The drawing under review shows one solid part. Ordinate dimensions are in mm from its lowest x, y, z. A direction names the side the tool comes from. Give positions to 0.01 mm unless a question says otherwise; leave off trailing zeros. Order: outer loops, then holes, each group sorted by start corner. A loop starts at its lowest first (then second) coordinate and runs counter-clockwise, first axis right, second up. Notation, with made-up numbers: (11, -18.5) -> (58, -18.5) arc R12 ccw to (58, -1.5) -> close; hole circle Ø4 at (3.5, -26.75). An arc over 180 degrees is marked (long way). Return JSON: item names as keys, results as strings. Group by question number.
1) To check wall thickness, follow line 1 along X through (y, z) = (1.75, 1.2); line 2 along X through (y, z) = (3.5, 1.5); line 3 along Z through (x, y) = (23.25, 4.25). State the ranges of each line that lie inside material, in increasing order.
2) The part is to be moulded in two halves that separate along X. For the marked faces 1, 2 and 3, say which applies: released by +X, released by -X, zero draft, split by the parting line, or undercut.
3) Add section D-D (y = 2). State how many separate pieces and enclosed holes the cut face has, then the cut area to 3 significant figures.
4) Insertion check: P1, Ø1.5, axis at x = 24.5, y = 5, coming from the +Z side; P2, Ø2, axis at x = 10.5, z = 1, coming from the -Y side (3 decimals); P3, Ø1.5, axis at x = 21, y = 5, coming from the +Z side. Each pin has a flat end and moves straight along its axis. Give the tip position at first contact, or say it passes through.
5) Add section B-B (z = 0.95). Give the boundary of the cut face in (x, y).
6) Add section A-A (x = 25.72). Give the boundary of the cut face in (y, z).
7) Add section C-C (y = 0.5). Give the boundary of the cut face in (x, z).
8) For the marked faces 4 and 5, list the 3-axis set-ups (+Z, -Z, +X, -X, +Y, -Y) from which the entire face can be reached by the end or side of a thin tool; tool diameter is ignored.
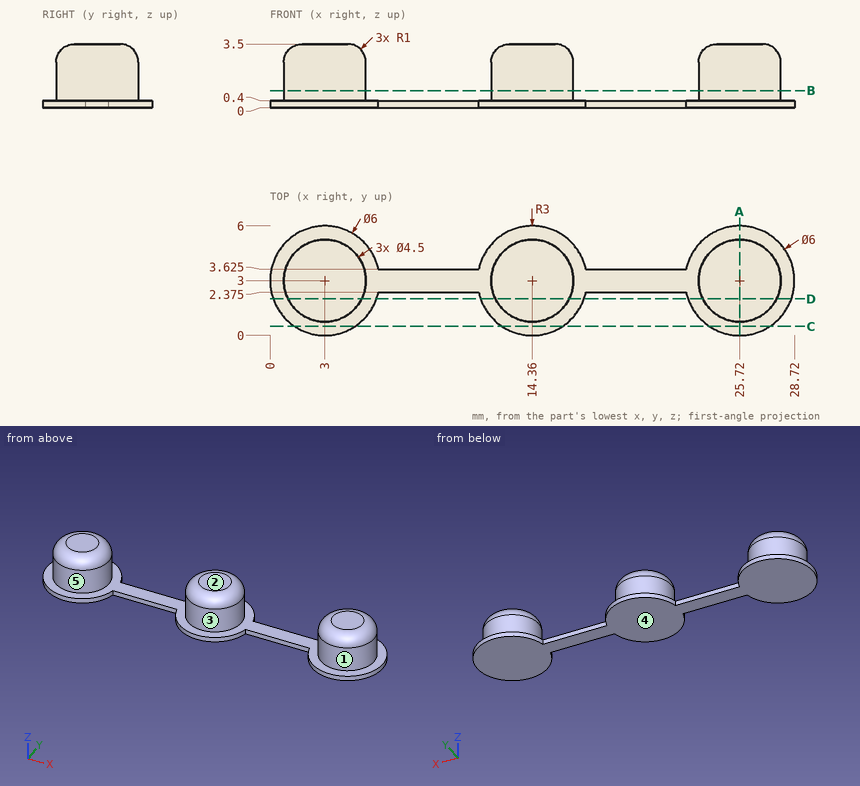
Evaluation:
{
 "1": {"line 1": "1.13 to 4.87, 12.49 to 16.23, 23.85 to 27.59", "line 2": "0.81 to 5.19, 12.17 to 16.55, 23.53 to 27.91", "line 3": "0 to 0.4"},
 "2": {"face 1": "undercut", "face 2": "zero draft", "face 3": "undercut"},
 "3": {"separate pieces": "3", "enclosed holes": "0", "area": "42.8 mm^2"},
 "4": {"P1": "z = 3.44", "P2": "y = 2.375", "P3": "through"},
 "5": {"outline": "circle Ø4.5 at (3, 3); circle Ø4.5 at (14.36, 3); circle Ø4.5 at (25.72, 3)"},
 "6": {"outline": "(0, 0) -> (6, 0) -> (6, 0.4) -> (5.25, 0.4) -> (5.25, 2.5) arc R1 ccw to (4.25, 3.5) -> (1.75, 3.5) arc R1 ccw to (0.75, 2.5) -> (0.75, 0.4) -> (0, 0.4) -> close"},
 "7": {"outline": "(1.34, 0) -> (4.66, 0) -> (4.66, 0.4) -> (1.34, 0.4) -> close; (12.7, 0) -> (16.02, 0) -> (16.02, 0.4) -> (12.7, 0.4) -> close; (24.06, 0) -> (27.38, 0) -> (27.38, 0.4) -> (24.06, 0.4) -> close"},
 "8": {"face 4": "-Z, +X, -X, +Y, -Y", "face 5": "+Z"}
}
